Read the model definition and answer for the solid it produces. Units are mm, in the model's axes. A direction names the side the tool comes from. Round coordinates to 2 decimals unless told otherwise and drop trailing zeros. Order: outer loops, then holes, each group sorted by start corner. A loop starts at its lowest first (then second) coordinate and runs counter-clockwise, first axis right, second up. Notation, with made-up numbers: (-34, 60.25) - (-6, 60.25) arc R27 ccw to (-6, 85.25) - close; hole circle Ø8 at (-4.75, 20.5). An arc over 180 degrees is marked (long way). Put each result on its own line as item: value. Start each with the question number.
Q1. Which of the six approach directions +Z, -Z, +X, -X, +Y, -Y give full straight-line access (tool end or side, diameter ignored) to faces 1 (the face through (22.66, -33.92, 14.01)), 2 (the face through (-3, 21, 10)), 3 (the face through (-3, -24.058, 5)), 4 (the face through (39, -34, 5.3))?
Q2. Section B-B on z = 16.25 is taken. Give the vertices of the cut face in (x, y).
Q3. Each of these flat-tipped pins is pushed along its axis until it touches: pin 1 Ø8 at (y, z) = (7, 11) entering from +X; pin 2 Ø1.8 at (x, y) = (43, -38) entering from +Z; pin 3 Ø1.6 at (x, z) = (30.5, 9) entering from +Y. Where does it stop, or does it pass through?
Q4. For a pull along Z with two mould halves and no side action, classify faces 5 (the face through (24.898, -33.918, 13.986)), 6 (the face through (36, -24.058, 19)), 7 (the face through (36, -31, 6.8)), 8 (the face through (36, -23, 10)) as pulls with the +Z half, pulls with the -Z half, needs draft (parallel to the pull), parting line crosses it, or undercut.
Q5. Section A-A on y = 5 is taken. Give the vertices of the cut face in (x, z), then the cut area to 3 significant figures.
Q6. Find the intervals of material crossed by line 1 along X through (y, z) = (43, 3); line 2 along Y through (x, z) = (35.5, 6.5); line 3 along Y through (x, z) = (21.5, 21.75), in increasing order. Write a range as from..to.
from build123d import *

# Parameters (mm, degrees)
SKETCH4_W           = 6
SKETCH4_H           = 100
BOSS_EXTRUDE2_DEPTH = 10
BOSS_EXTRUDE3_DEPTH = 80
SKETCH6_W           = 86
SKETCH6_H           = 20
BOSS_EXTRUDE4_DEPTH = 3
SKETCH7_R           = 1.026650489
CUT_EXTRUDE2_DEPTH  = 10
BOSS_EXTRUDE6_DEPTH = 20
CUT_EXTRUDE3_DEPTH  = 10
SKETCH11_W          = 86
SKETCH11_H          = 10
BOSS_EXTRUDE7_DEPTH = 15


with BuildPart() as part:
    # Sketch4 → Boss-Extrude2 (new body)
    with BuildSketch(Plane.XY):
        with Locations((-3, 5.941704036)):
            Rectangle(SKETCH4_W, SKETCH4_H)
    extrude(amount=BOSS_EXTRUDE2_DEPTH)

    # Sketch5 → Boss-Extrude3 (add)
    with BuildSketch(Plane(origin=(0, 0, 0), x_dir=(0, 0, -1), z_dir=(1, 0, 0))):
        Polygon((-10, -32.758295964), (-6.8, -32.758295964), (-6.8, -29.358295964), (-5.3, -29.358295964), (-5.3, -38.958295964), (-6.8, -38.958295964), (-6.8, -35.558295964), (-10, -35.558295964), align=None)
    extrude(amount=BOSS_EXTRUDE3_DEPTH)

    # Sketch6 → Boss-Extrude4 (add)
    with BuildSketch(Plane.XY.offset(10)):
        with Locations((37, -34.058295964)):
            Rectangle(SKETCH6_W, SKETCH6_H)
    extrude(amount=BOSS_EXTRUDE4_DEPTH)

    # Sketch7 → Cut-Extrude2 (cut)
    with BuildSketch(Plane(origin=(0, -35.558295964, 0), x_dir=(-1, 0, 0), z_dir=(0, -1, 0))):
        with Locations((-78.362195551, -8.533372311)):
            Circle(SKETCH7_R)
    extrude(amount=-CUT_EXTRUDE2_DEPTH, mode=Mode.SUBTRACT)

    # Sketch8 → Boss-Extrude6 (add)
    with BuildSketch(Plane(origin=(0, -24.058295964, 0), x_dir=(1, 0, 0), z_dir=(0, 1, 0))):
        Polygon((80, -13), (77.763932023, -15), (75.527864045, -13), align=None)
        Polygon((75.5, -13), (73.263932023, -15), (71.027864045, -13), align=None)
        Polygon((71, -13), (68.763932023, -15), (66.527864045, -13), align=None)
        Polygon((66.5, -13), (64.263932023, -15), (62.027864045, -13), align=None)
        Polygon((62, -13), (59.763932023, -15), (57.527864045, -13), align=None)
        Polygon((57.5, -13), (55.263932023, -15), (53.027864045, -13), align=None)
        Polygon((53, -13), (50.763932023, -15), (48.527864045, -13), align=None)
        Polygon((48.5, -13), (46.263932023, -15), (44.027864045, -13), align=None)
        Polygon((44, -13), (41.763932023, -15), (39.527864045, -13), align=None)
        Polygon((39.5, -13), (37.263932023, -15), (35.027864045, -13), align=None)
        Polygon((35, -13), (32.763932023, -15), (30.527864045, -13), align=None)
        Polygon((30.5, -13), (28.263932023, -15), (26.027864045, -13), align=None)
        Polygon((26, -13), (23.763932023, -15), (21.527864045, -13), align=None)
        Polygon((21.5, -13), (19.263932023, -15), (17.027864045, -13), align=None)
        Polygon((17, -13), (14.763932023, -15), (12.527864045, -13), align=None)
        Polygon((12.5, -13), (10.263932023, -15), (8.027864045, -13), align=None)
        Polygon((8, -13), (5.763932023, -15), (3.527864045, -13), align=None)
        Polygon((3.5, -13), (1.263932023, -15), (-0.972135955, -13), align=None)
        Polygon((-1, -13), (-3.236067977, -15), (-5.472135955, -13), align=None)
    extrude(amount=-BOSS_EXTRUDE6_DEPTH)

    # Sketch9 → Cut-Extrude3 (cut)
    with BuildSketch(Plane(origin=(0, 0, 0), x_dir=(0, 0, -1), z_dir=(1, 0, 0))):
        Polygon((-10, -24.058295964), (3.159373841, -24.058295964), (3.159373841, -44.058295964), (-10, -44.058295964), (-10, -35.558295964), (-6.8, -35.558295964), (-6.8, -39.06749372), (-5.2003516, -39.06749372), (-5.2003516, -29.455913505), (-6.8, -29.455913505), (-6.8, -32.758295964), (-10, -32.758295964), align=None)
    extrude(amount=-CUT_EXTRUDE3_DEPTH, mode=Mode.SUBTRACT)

    # Sketch11 → Boss-Extrude7 (add)
    with BuildSketch(Plane.XY.offset(10)):
        with Locations((37, -19.058295964)):
            Rectangle(SKETCH11_W, SKETCH11_H)
    extrude(amount=BOSS_EXTRUDE7_DEPTH)


solid = part.part
Findings:
1. face 1: +Z, -Y
1. face 2: +Z, +X, -X, +Y
1. face 3: -Z, +X, -X
1. face 4: -Z, +X, +Y, -Y
2. outline: (-6, -24.06) - (80, -24.06) - (80, -14.06) - (-6, -14.06) - close
3. pin 1: x = 0
3. pin 2: z = 14.7
3. pin 3: y = -32.76
4. face 5: pulls with the +Z half
4. face 6: needs draft
4. face 7: undercut
4. face 8: undercut
5. outline: (-6, 0) - (0, 0) - (0, 10) - (-6, 10) - close
5. area: 60.0 mm2
6. line 1: -6..0
6. line 2: -38.96..-29.36
6. line 3: -24.06..-14.06
